Verification items for the finished model (mm, model axes). Face numbers are marked on the shaded views. Round coordinates to 2 decimals unless told otherwise and drop trailing zeros. Order: outer loops, then holes, each group sorted by start corner. A loop starts at its lowest first (then second) coordinate and runs counter-clockwise, first axis right, second up. Notation, with made-up numbers: (85.25, 84) -> (109.25, 84) arc R26 ccw to (109.25, 104) -> close; hole circle Ø7 at (33.25, 57.5). An arc over 180 degrees is marked (long way). Put each result on its own line as item: value.
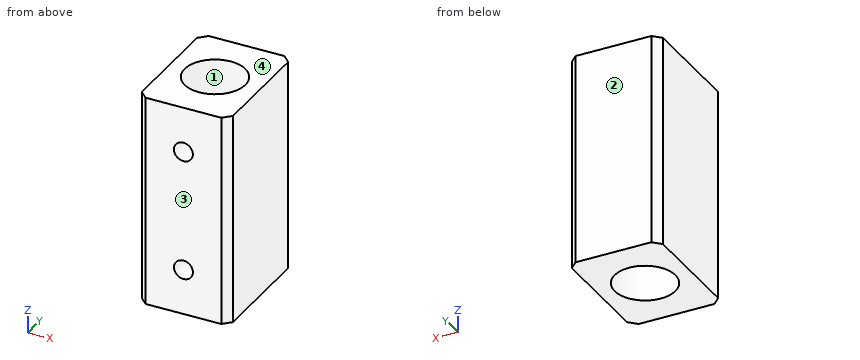
from build123d import *

# Parameters (mm, degrees)
ESQUISSE1_W           = 12
ESQUISSE1_H           = 16
ESQUISSE1_R           = 4
BOSS_EXTRU_1_DEPTH    = 14
CHANFREIN1_SIZE       = 1
TROU_TARAUD_M31_D     = 2.5
TROU_TARAUD_M31_DEPTH = 8.5
TROU_TARAUD_M31_TIP   = 0.751075774


with BuildPart() as part:
    # Esquisse1 → Boss.-Extru.1 (new, symmetric)
    with BuildSketch(Plane.XY):
        Rectangle(ESQUISSE1_W, ESQUISSE1_H)
        Circle(ESQUISSE1_R, mode=Mode.SUBTRACT)
    extrude(amount=BOSS_EXTRU_1_DEPTH, both=True)

    # Chanfrein1
    chanfrein1_edges = [part.edges().sort_by_distance(p)[0] for p in [
        (-6, 8, 0),
        (6, 8, 0),
        (6, -8, 0),
        (-6, -8, 0),
    ]]
    chamfer(chanfrein1_edges, length=CHANFREIN1_SIZE)

    # Trou taraudé M31
    with Locations(Plane(origin=(0, -8, 0), x_dir=(-1, 0, 0), z_dir=(0, -1, 0))):
        with Locations((0, 8), (0, -8)):
            Hole(TROU_TARAUD_M31_D / 2, depth=TROU_TARAUD_M31_DEPTH)
            with Locations((0, 0, -(TROU_TARAUD_M31_DEPTH + TROU_TARAUD_M31_TIP / 2))):  # 118° drill point
                Cone(0, TROU_TARAUD_M31_D / 2, TROU_TARAUD_M31_TIP, mode=Mode.SUBTRACT)


solid = part.part
Item 1: Section check D-D on z = 8. Record the boundary of the cut face in (x, y), then the cut area to 3 significant figures.
Check sheet entries:
outline: (-6, -7) -> (-5, -8) -> (-1.25, -8) -> (-1.25, -3.8) arc R4 cw (long way) to (1.25, -3.8) -> (1.25, -8) -> (5, -8) -> (6, -7) -> (6, 7) -> (5, 8) -> (-5, 8) -> (-6, 7) -> close
area: 130 mm^2
Item 2: Section check A-A on x = 0. Record the boundary of the cut face in (y, z).
Check sheet entries:
outline: (-8, -14) -> (-4, -14) -> (-4, -9.25) -> (-8, -9.25) -> close; (-8, -6.75) -> (-4, -6.75) -> (-4, 6.75) -> (-8, 6.75) -> close; (-8, 9.25) -> (-4, 9.25) -> (-4, 14) -> (-8, 14) -> close; (4, -14) -> (8, -14) -> (8, 14) -> (4, 14) -> close
Item 3: Section check B-B on y = 0. Record the boundary of the cut face in (x, z), then the cut area to 3 significant figures.
Check sheet entries:
outline: (-6, -14) -> (-4, -14) -> (-4, 14) -> (-6, 14) -> close; (4, -14) -> (6, -14) -> (6, 14) -> (4, 14) -> close
area: 112 mm^2
Item 4: Release check for a two-part mould opening along Y. For the marked faces 1, 2, 3 and 4 record: +Y half, -Y half, draft (parallel to the pull), parting line (faces both ways), or undercut.
Check sheet entries:
face 1: undercut
face 2: +Y half
face 3: -Y half
face 4: draft
Item 5: Material ranges on L1, parallel to Z at x = 0, y = -6.5; L2, parallel to X at y = -6.4, z = 8; L3, parallel to X at y = -7.1, z = -8, recorded low to high. Write a range as [from, to].
Check sheet entries:
L1: z = [-14, -9.25], [-6.75, 6.75], [9.25, 14]
L2: x = [-6, -1.25], [1.25, 6]
L3: x = [-5.9, -1.25], [1.25, 5.9]
Item 6: Gauge pin test, flat ends, axial feed: pin 1 Ø6.5 at (x, y) = (0, 0) entering from -Z; pin 2 Ø2 at (x, z) = (0, 8) entering from -Y. Record the tip position at first contact, or that the pin passes through.
Check sheet entries:
pin 1: passes through
pin 2: stops at y = 3.87
Item 7: Section check C-C on z = -0.75. Record the boundary of the cut face in (x, y), then the cut area to 3 significant figures.
Check sheet entries:
outline: (-6, -7) -> (-5, -8) -> (5, -8) -> (6, -7) -> (6, 7) -> (5, 8) -> (-5, 8) -> (-6, 7) -> close; hole circle Ø8 at (0, 0)
area: 140 mm^2
